from build123d import *

# Parameters (mm, degrees)
F0_R          = 10.033
F1_DEPTH      = 219.075
F3_W          = 39.878
F3_H          = 74.93
F4_DEPTH      = 127
F5_W          = 39.878
F5_H          = 40.005
F6_DEPTH      = 22.225
F7_R          = 3.937
F8_DEPTH      = 55.881
F8_DEPTH_BACK = 19.051


with BuildPart() as f1:
    # F0 (on Right) → F1 (new body)
    with BuildSketch(Plane.YZ):
        Circle(F0_R)
    extrude(amount=F1_DEPTH)

    # F3 (on offset) → F4 (join)
    with BuildSketch(Plane.YZ.offset(19.05)):
        with Locations((0, -18.415)):
            Rectangle(F3_W, F3_H)
    extrude(amount=F4_DEPTH)

    # F5 (on face) → F6 (cut)
    with BuildSketch(Plane.YZ.offset(146.05)):
        with Locations((0, -35.8775)):
            Rectangle(F5_W, F5_H)
    extrude(amount=-F6_DEPTH, mode=Mode.SUBTRACT)

    # F7 (on Top) → F8 (cut, two sides)
    with BuildSketch(Plane.XY) as f8_sk:
        with Locations((6.35, 0)):
            Circle(F7_R)
        with Locations((212.852, 0)):
            Circle(F7_R)
    extrude(amount=-F8_DEPTH, mode=Mode.SUBTRACT)
    extrude(f8_sk.sketch, amount=F8_DEPTH_BACK, mode=Mode.SUBTRACT)


solid = f1.part
Model file for the job. Use its own axes, mm. A direction names the side the tool comes from. Give positions to 0.01 mm unless a question says otherwise; leave off trailing zeros. Write each loop counter-clockwise with the first axis right and the second up, starting at its lowest first coordinate (ties: lowest second). Pieces come first, ordered by that corner, then holes. Notation, with made-up numbers: (-13, 40.5) -> (23, 40.5) arc R31 cw to (23, 79.5) -> close; hole circle Ø11 at (22, 72). An arc over 180 degrees is marked (long way). Write item = value, one per line.
(1) Tool access for faces 1 (the face through (146.05, -5, 10)), 2 (the face through (123.825, 0, -36)), 3 (the face through (9.39, 9.27, -3.84)): list every direction of +Z, -Z, +X, -X, +Y, -Y with a clear straight run to the whole face (end or side of a thin tool).
Determined:
face_1 = +X
face_2 = -Z, +X, +Y, -Y
face_3 = -X
(2) Flat gauge pins, fed straight in: P1, Ø4, axis at y = -4.5, z = -35, coming from the +X side (3 decimals); P2, Ø4, axis at y = -5, z = -16, coming from the +X side; P3, Ø10, axis at x = 6.35, y = 0, coming from the +Z side. Where does each tip first touch, or does it go through?
Determined:
P1 = 123.825
P2 = 146.05
P3 = 10.03
(3) Probe line 1 along X through (y, z) = (0, 3) (3 decimals); line 2 along Z through (x, y) = (126, -1) (3 decimals); line 3 along X through (y, z) = (-9, -24) (3 decimals). List the from-to ranges inside material, lowest first.
Determined:
line_1 = 0 to 2.413, 10.287 to 208.915, 216.789 to 219.075
line_2 = -15.875 to 19.05
line_3 = 19.05 to 123.825
(4) Slice it at B-B, the plane z = -3. Give the cut face in (x, y) (3 decimals).
Determined:
outline = (0, -9.574) -> (19.05, -9.574) -> (19.05, -19.939) -> (146.05, -19.939) -> (146.05, -9.574) -> (219.075, -9.574) -> (219.075, 9.574) -> (146.05, 9.574) -> (146.05, 19.939) -> (19.05, 19.939) -> (19.05, 9.574) -> (0, 9.574) -> close; hole circle Ø7.874 at (6.35, 0); hole circle Ø7.874 at (212.852, 0)
(5) Slice it at C-C, the plane y = -15. Give the cut face in (x, z) (3 decimals), then the cut area to 3 significant figures.
Determined:
outline = (19.05, -55.88) -> (123.825, -55.88) -> (123.825, -15.875) -> (146.05, -15.875) -> (146.05, 19.05) -> (19.05, 19.05) -> close
area = 8,630 mm2
(6) Slice it at A-A, the plane y = 0. Give the cut face in (x, z) (3 decimals).
Determined:
outline = (0, -10.033) -> (2.413, -10.033) -> (2.413, 10.033) -> (0, 10.033) -> close; (10.287, -10.033) -> (19.05, -10.033) -> (19.05, -55.88) -> (123.825, -55.88) -> (123.825, -15.875) -> (146.05, -15.875) -> (146.05, -10.033) -> (208.915, -10.033) -> (208.915, 10.033) -> (146.05, 10.033) -> (146.05, 19.05) -> (19.05, 19.05) -> (19.05, 10.033) -> (10.287, 10.033) -> close; (216.789, -10.033) -> (219.075, -10.033) -> (219.075, 10.033) -> (216.789, 10.033) -> close
(7) Slice it at D-D, the plane x = 6.35. Give the cut face in (y, z).
Determined:
outline = (-3.94, -9.23) -> (-3.94, 9.23) arc R10.03 ccw to start; (3.94, -9.23) arc R10.03 ccw to (3.94, 9.23) -> close
